For this review, take the finished solid that the model builds, in its own axes (mm). A direction names the side the tool comes from. Give positions to 0.01 mm unless a question says otherwise; leave off trailing zeros. Loops run counter-clockwise (first coordinate to the right, second up) from the corner with the lowest first, then second, coordinate; pieces in that order, holes last.
```python
from build123d import *

# Parameters (mm, degrees)
SKETCH1_W           = 16
SKETCH1_H           = 48.5
BOSS_EXTRUDE1_DEPTH = 7
SKETCH2_W           = 5.4
SKETCH2_H           = 3.7
CUT_EXTRUDE1_DEPTH  = 27.47758486
SKETCH3_OUTSIDE_W   = 28.31
SKETCH3_OUTSIDE_H   = 19.31
SKETCH3_OUTSIDE_W_2 = 16
SKETCH3_OUTSIDE_H_2 = 7
SKETCH3_OUTSIDE_R   = 1.5
CUT_EXTRUDE2_DEPTH  = 11
SKETCH4_W           = 16
SKETCH4_H           = 20
CUT_EXTRUDE3_DEPTH  = 3
CHAMFER1_SIZE       = 3
SKETCH5_W           = 2
SKETCH5_H           = 7.7
BOSS_EXTRUDE2_DEPTH = 7
CHAMFER2_SIZE       = 2
CHAMFER3_SIZE       = 1


with BuildPart() as part:
    # Sketch1 → Boss-Extrude1 (new body)
    with BuildSketch(Plane.XY):
        Rectangle(SKETCH1_W, SKETCH1_H)
    extrude(amount=BOSS_EXTRUDE1_DEPTH)

    # Sketch2 → Cut-Extrude1 (cut, through all)
    with BuildSketch(Plane.XY.offset(7)):
        with Locations((-4, 16.1)):
            Rectangle(SKETCH2_W, SKETCH2_H)
        with Locations((4, 16.1)):
            Rectangle(SKETCH2_W, SKETCH2_H)
        with Locations((4, -14.1)):
            Rectangle(SKETCH2_W, SKETCH2_H)
        with Locations((-4, -14.1)):
            Rectangle(SKETCH2_W, SKETCH2_H)
    extrude(amount=-CUT_EXTRUDE1_DEPTH, mode=Mode.SUBTRACT)

    # Sketch3 outside → Cut-Extrude2 (cut)
    # profile 1 of 3: a face of its own
    with BuildSketch(Plane(origin=(0, 24.25, 0), x_dir=(1, 0, 0), z_dir=(0, 1, 0))):
        with Locations((0, -3.5)):
            Rectangle(SKETCH3_OUTSIDE_W, SKETCH3_OUTSIDE_H)
        with Locations((0, -3.5)):
            Rectangle(SKETCH3_OUTSIDE_W_2, SKETCH3_OUTSIDE_H_2, mode=Mode.SUBTRACT)
    # profile 2 of 3: a face of its own
    with BuildSketch(Plane(origin=(0, 24.25, 0), x_dir=(1, 0, 0), z_dir=(0, 1, 0))):
        with Locations(Location((4, -3.5, 0), (0, 0, 270))):
            Circle(SKETCH3_OUTSIDE_R)
    # profile 3 of 3: a face of its own
    with BuildSketch(Plane(origin=(0, 24.25, 0), x_dir=(1, 0, 0), z_dir=(0, 1, 0))):
        with Locations(Location((-4, -3.5, 0), (0, 0, 270))):
            Circle(SKETCH3_OUTSIDE_R)
    cut_extrude2 = extrude(amount=-CUT_EXTRUDE2_DEPTH, mode=Mode.SUBTRACT)

    # Mirror1: Cut-Extrude2 across plane
    add(cut_extrude2.mirror(Plane.ZX), mode=Mode.SUBTRACT)

    # Sketch4 → Cut-Extrude3 (cut)
    with BuildSketch(Plane.XY.offset(7)):
        Rectangle(SKETCH4_W, SKETCH4_H)
    extrude(amount=-CUT_EXTRUDE3_DEPTH, mode=Mode.SUBTRACT)

    # Chamfer1
    chamfer1_edges = [part.edges().sort_by_distance(p)[0] for p in [
        (0, -10, 4),
        (0, 10, 4),
    ]]
    chamfer(chamfer1_edges, length=CHAMFER1_SIZE - 0.0001)  # a hair under: the kernel refuses the full size

    # Sketch5 → Boss-Extrude2 (add)
    with BuildSketch(Plane(origin=(0, 0, 0), x_dir=(-1, 0, 0), z_dir=(0, 0, -1))):
        with Locations((9, 16.1)):
            Rectangle(SKETCH5_W, SKETCH5_H)
        with Locations((-9, 16.1)):
            Rectangle(SKETCH5_W, SKETCH5_H)
        with Locations((-9, -14.1)):
            Rectangle(SKETCH5_W, SKETCH5_H)
        with Locations((9, -14.1)):
            Rectangle(SKETCH5_W, SKETCH5_H)
    extrude(amount=-BOSS_EXTRUDE2_DEPTH)

    # Chamfer2
    chamfer2_edges = [part.edges().sort_by_distance(p)[0] for p in [
        (-10, -17.95, 3.5),
        (-10, -10.25, 3.5),
        (10, -17.95, 3.5),
        (10, -10.25, 3.5),
        (10, 12.25, 3.5),
        (10, 19.95, 3.5),
        (-10, 12.25, 3.5),
        (-10, 19.95, 3.5),
    ]]
    chamfer(chamfer2_edges, length=CHAMFER2_SIZE - 0.0001)  # a hair under: the kernel refuses the full size

    # Chamfer3
    chamfer3_edges = [part.edges().sort_by_distance(p)[0] for p in [
        (-6.7, -12.25, 3.5),
        (-1.3, -12.25, 3.5),
        (6.7, -12.25, 3.5),
        (1.3, -12.25, 3.5),
        (6.7, 14.25, 3.5),
        (1.3, 14.25, 3.5),
        (-1.3, 14.25, 3.5),
        (-6.7, 14.25, 3.5),
    ]]
    chamfer(chamfer3_edges, length=CHAMFER3_SIZE)


solid = part.part
```
Q1. Consider section B-B on y = -19.5. Give the boundary of the cut face in (x, z), plus the area to 3 significant figures.
Answers:
outline: (-8, 0) - (8, 0) - (8, 7) - (-8, 7) - close; hole circle Ø3 at (-4, 3.5); hole circle Ø3 at (4, 3.5)
area: 97.9 mm2
Q2. For pin 1 Ø11 at (x, y) = (-2, 2.5) entering from +Z; pin 2 Ø2 at (y, z) = (5.5, 1) entering from +X; pin 3 Ø10 at (x, y) = (-2, 1.5) entering from +Z, all flat-tipped, find the tip position at first contact; note any pin that passes through.
Answers:
pin 1: stops at z = 5
pin 2: stops at x = 8
pin 3: stops at z = 4
Q3. Consider section A-A on x = -4. Count the separate pieces of the cut face and the enclosed holes in it, plus the area to 3 significant figures.
Answers:
separate pieces: 5
enclosed holes: 0
area: 190 mm2
Q4. Machinability: for faces 1 (the flat face through (9.01, 18.94, 3.45)), 2 (the flat face through (6.7, -15, 4)), 3 (the flat face through (-8, 22, 3)), 4 (the cylindrical face through (-4, -20, 5)), which of the approach directions +Z, -Z, +X, -X, +Y, -Y give a long, thin tool a straight path to every point of the face, cutting with its end or side? Answer none if there is none.
Answers:
face 1: +Z, -Z, +X, +Y
face 2: +Z, -Z
face 3: +Z, -Z, -X, +Y
face 4: -Y
Q5. Mouldability with a two-part tool opening along Z and no side actions: class faces 5 (the cylindrical face through (4, 21, 5)), 6 (the flat face through (0, 17, 7)), 7 (the flat face through (-6.21, 14.76, 3.55)), 8 (the cylindrical face through (4, 14, 5)) as +Z half, -Z half, draft (parallel to the pull), parting line (faces both ways), or undercut.
Answers:
face 5: undercut
face 6: +Z half
face 7: draft
face 8: undercut
Q6. For probe 1 along X at (y, z) = (-20, 3.5); probe 2 along Y at (x, z) = (2.5, 1.5); probe 3 along Z at (x, y) = (4, -19.25), list the stretches that pass through material, from the lowest coordinate up.
Answers:
probe 1: x = -8 to -5.5, -2.5 to 2.5, 5.5 to 8
probe 2: y = -24.25 to -15.95, -12.25 to 14.25, 17.95 to 24.25
probe 3: z = 0 to 2, 5 to 7
